For this review, take the finished solid that the model builds, in its own axes (mm). A direction names the side the tool comes from. Round coordinates to 2 decimals unless told otherwise and drop trailing zeros. Loops run counter-clockwise (first coordinate to the right, second up) from the corner with the lowest first, then second, coordinate; pieces in that order, holes last. Notation, with made-up numbers: M -24.75,80.5 L 16.25,80.5 A34 ccw 16.25,114.5 Z; hole C 25.25,37 d5. An arc over 180 degrees is marked long. One line per question, with ' | ' between items. Start each with the question number.
1) We need section D-D (x = -12.5). Give the boundary of the cut face in (y, z), and give its area (3 significant figures).
2) For pin 1 Ø1.3 at (x, y) = (253, -70.5) entering from -Z; pin 2 Ø3 at (y, z) = (-52, 1.5) entering from +X; pin 3 Ø1.5 at (x, y) = (-4.5, -52) entering from +Z, all flat-tipped, find the tip position at first contact; note any pin that passes through.
3) We need section A-A (y = -54). Give the boundary of the cut face in (x, z).
4) For probe 1 along X at (y, z) = (-13, 80); probe 2 along Y at (x, z) = (13, 27.5); probe 3 along X at (y, z) = (-46, 78.5), list the stretches that pass through material, from the lowest coordinate up. Write a range as from..to.
5) Mouldability with a two-part tool opening along X and no side actions: class faces 4 (the face through (-4, 2, 0)), 5 (the face through (251.46, -2, 103)), 6 (the face through (-4, 2, 2.54)), 7 (the face through (254, -2, 101)) as pulls with the +X half, pulls with the -X half, needs draft (parallel to the pull), parting line crosses it, or undercut.
6) We need section B-B (z = 184.5). Give the boundary of the cut face in (x, y), and give its area (3 significant figures).
7) We need section C-C (y = -7). Give the boundary of the cut face in (x, z).
8) For faces 1 (the face through (252, -90.686, 40)), 2 (the face through (4, 127, 101)), 3 (the face through (-251.46, -2, 103)), list the 3-axis set-ups (+Z, -Z, +X, -X, +Y, -Y) from which the entire face can be reached by the end or side of a thin tool; tool diameter is ignored.
```python
from build123d import *

# Parameters (mm, degrees)
F0_W     = 508
F0_H     = 254
F1_DEPTH = 2.54
F2_W     = 505.46
F2_H     = 2.54
F3_DEPTH = 203.2
F4_W     = 2.54
F4_H     = 248.92
F5_DEPTH = 203.2
F6_W     = 54.724466
F6_H     = 102.87
F7_DEPTH = 25.4


with BuildPart() as f1:
    # F0 (on Top) → F1 (new body)
    with BuildSketch(Plane.XY):
        Rectangle(F0_W, F0_H)
    extrude(amount=F1_DEPTH)

    # F2 (on face) → F3 (join)
    with BuildSketch(Plane.XY.offset(2.54)):
        Polygon((-251.46, 127), (-254, 127), (-254, -127), (-251.46, -127), (-251.46, 124.46), align=None)
        with Locations((1.27, 125.73)):
            Rectangle(F2_W, F2_H)
    extrude(amount=F3_DEPTH)

    # F4 (on face) → F5 (join)
    with BuildSketch(Plane.XY.offset(2.54)):
        Polygon((-251.46, -124.46), (-251.46, -127), (254, -127), (254, -124.46), (251.46, -124.46), align=None)
        with Locations((252.73, 0)):
            Rectangle(F4_W, F4_H)
    extrude(amount=F5_DEPTH)

    # F6 (on face) → F7 (cut)
    with BuildSketch(Plane.YZ.offset(254)):
        with Locations((-63.324029, 51.435)):
            Rectangle(F6_W, F6_H)
    extrude(amount=-F7_DEPTH, mode=Mode.SUBTRACT)


solid = f1.part
```
Answers below:
1) outline: M -127,0 L 127,0 L 127,205.74 L 124.46,205.74 L 124.46,2.54 L -124.46,2.54 L -124.46,205.74 L -127,205.74 Z | area: 1,680 mm^2
2) pin 1: z = 102.87 | pin 2: x = 228.6 | pin 3: z = 2.54
3) outline: M -254,0 L 228.6,0 L 228.6,2.54 L -251.46,2.54 L -251.46,205.74 L -254,205.74 Z; M 251.46,102.87 L 254,102.87 L 254,205.74 L 251.46,205.74 Z
4) probe 1: -254..-251.46, 251.46..254 | probe 2: -127..-124.46, 124.46..127 | probe 3: -254..-251.46
5) face 4: needs draft | face 5: undercut | face 6: undercut | face 7: pulls with the +X half
6) outline: M -254,-127 L 254,-127 L 254,127 L -254,127 Z; hole M -251.46,-124.46 L 251.46,-124.46 L 251.46,124.46 L -251.46,124.46 Z | area: 3,850 mm^2
7) outline: M -254,0 L 254,0 L 254,205.74 L 251.46,205.74 L 251.46,2.54 L -251.46,2.54 L -251.46,205.74 L -254,205.74 Z
8) face 1: -Z, +X | face 2: +Z, -Z, +X, -X, +Y | face 3: +Z
